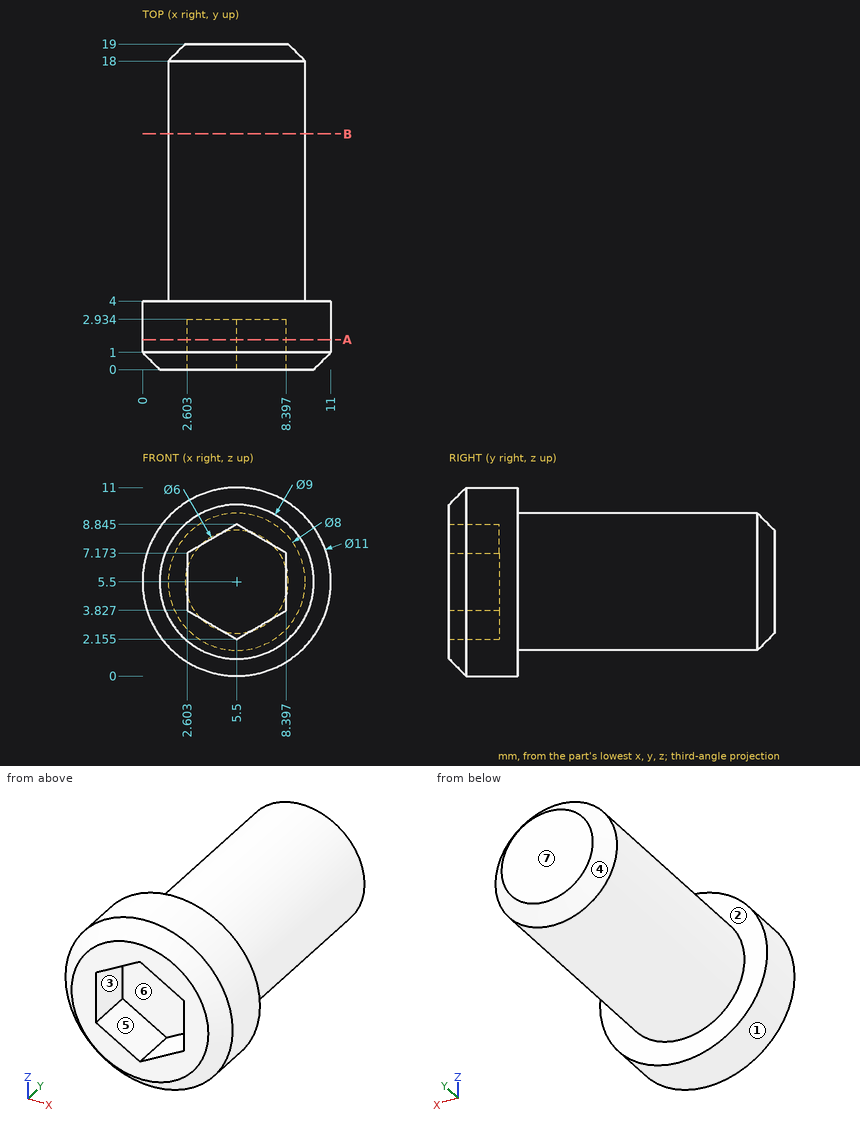
Verification items for this drawing (mm, ordinates from the low corner). A direction names the side the tool comes from. Round coordinates to 2 decimals unless told otherwise and drop trailing zeros. Order: outer loops, then holes, each group sorted by start corner. A loop starts at its lowest first (then second) coordinate and runs counter-clockwise, first axis right, second up.
1) Depth check by flat-ended pin: pin 1 (1 mm diameter, centred on x = 3, z = 2, fed in from +Y); pin 2 (3 mm diameter, centred on y = 15, z = 4, fed in from -X); pin 3 (1 mm diameter, centred on x = 3.5, y = 15, fed in from +Z). Enter the tip coordinate at first touch or a pass-through.
Geometry says:
pin 1: stops at y = 18.2
pin 2: stops at x = 1.5
pin 3: stops at z = 9.21
2) Tool access check on the marked faces 1, 2 and 3. Record the directions out of +Z, -Z, +X, -X, +Y, -Y that give a thin tool (end or side, any length) a straight path to the whole face; none if there is none.
Geometry says:
face 1: +Y, -Y
face 2: +Y
face 3: -Y
3) Draft check along Z on the marked faces 4, 5, 6 and 7. Enter one of: +Z half, -Z half, draft (parallel to the pull), parting line (faces both ways), or undercut.
Geometry says:
face 4: parting line
face 5: undercut
face 6: undercut
face 7: draft
4) Cross-section at B-B, the plane y = 13.75. Record the cut outline in (x, z).
Geometry says:
outline: circle Ø8 at (5.5, 5.5)
5) Cross-section at A-A, the plane y = 1.75. Record the cut outline in (x, z) (1 decimal).
Geometry says:
outline: circle Ø11 at (5.5, 5.5); hole (2.6, 3.8) - (5.5, 2.2) - (8.4, 3.8) - (8.4, 7.2) - (5.5, 8.8) - (2.6, 7.2) - close
6) Material ranges on line 1 (Z direction, x = 5.5, y = 16.25); line 2 (Y direction, x = 8, z = 2.25); line 3 (Y direction, x = 7.75, z = 6.5) (1 decimal), recorded low to high.
Geometry says:
line 1: z = 1.5 to 9.5
line 2: y = 0 to 4
line 3: y = 2.9 to 19
